```python
from build123d import *

# Parameters (mm, degrees)
F1_DEPTH = 40.2336
F2_DEPTH = 15.7734
F3_R     = 3.302


# Not quite as in the source:
# - a feature names something its author has since deleted; it is built from what else it names


with BuildPart() as f1:
    # F0 (on Top) → F1 (new body)
    with BuildSketch(Plane.XY):
        with BuildLine():
            ThreePointArc((5.2118165727, -28.0956863773), (21.9710978739, -18.2702348977), (28.575, 0))
            ThreePointArc((28.575, 0), (21.9710978739, 18.2702348977), (5.2118165727, 28.0956863773))
            ThreePointArc((5.2118165727, 28.0956863773), (-28.575, 0), (5.2118165727, -28.0956863773))
        make_face()
        with BuildLine():
            ThreePointArc((13.4477648793, -4.826), (-14.2875, 0), (13.4477648793, 4.826))
            Line((13.4477648793, 4.826), (19.7977648793, 4.826))
            Line((19.7977648793, 4.826), (19.7977648793, 0))
            Line((19.7977648793, 0), (19.7977648793, -4.826))
            Line((19.7977648793, -4.826), (13.4477648793, -4.826))
        make_face(mode=Mode.SUBTRACT)
    extrude(amount=F1_DEPTH)

    # F0 (on Top) → F2 (join)
    with BuildSketch(Plane.XY):
        with BuildLine():
            ThreePointArc((5.2118165727, 28.0956863773), (21.9710978739, 18.2702348977), (28.575, 0))
            Line((28.575, 0), (34.925, 0))
            ThreePointArc((34.925, 0), (40.5046158184, 13.4703841816), (53.975, 19.05))
            Line((53.975, 19.05), (5.2118165727, 28.0956863773))
        make_face()
        with BuildLine():
            Line((34.925, 0), (28.575, 0))
            ThreePointArc((28.575, 0), (21.9710978739, -18.2702348977), (5.2118165727, -28.0956863773))
            Line((5.2118165727, -28.0956863773), (53.975, -19.05))
            ThreePointArc((53.975, -19.05), (40.5046158184, -13.4703841816), (34.925, 0))
        make_face()
        with BuildLine():
            ThreePointArc((53.975, 19.05), (40.5046158184, 13.4703841816), (34.925, 0))
            ThreePointArc((34.925, 0), (40.5046158184, -13.4703841816), (53.975, -19.05))
            ThreePointArc((53.975, -19.05), (67.4453841816, -13.4703841816), (73.025, 0))
            ThreePointArc((73.025, 0), (67.4453841816, 13.4703841816), (53.975, 19.05))
        make_face()
        with BuildLine():
            ThreePointArc((64.135, 0), (53.975, -10.16), (43.815, 0))
            ThreePointArc((43.815, 0), (53.975, 10.16), (64.135, 0))
        make_face(mode=Mode.SUBTRACT)
    extrude(amount=F2_DEPTH)

    # F3
    f3_edges = [f1.edges().sort_by_distance(p)[0] for p in [
        (-5.211817, 28.095686, 40.2336),
    ]]
    fillet(f3_edges, radius=F3_R)


solid = f1.part
```
Read the model definition and answer for the solid it produces. Units are mm, in the model's axes. A direction names the side the tool comes from. Coordinates: 2 decimals unless noted, no trailing zeros. Write each loop counter-clockwise with the first axis right and the second up, starting at its lowest first coordinate (ties: lowest second). Pieces come first, ordered by that corner, then holes. Notation, with made-up numbers: (80.25, 77) - (89.25, 77) arc R30 cw to (89.25, 108) - close; hole circle Ø10 at (67.5, -15). An arc over 180 degrees is marked (long way). Answer as a JSON object with one key per item and string values. Group by question number.
1. Which of the six approach directions +Z, -Z, +X, -X, +Y, -Y give full straight-line access (tool end or side, diameter ignored) to faces 4 (the flat face through (22, 0, 0)), 5 (the flat face through (19.798, 0, 20))?
2. Consider L1, parallel to Y at x = 0, z = 22 (1 decimal); L2, parallel to X at y = 0, z = 18 (1 decimal); L3, parallel to X at y = 3, z = 15.5. Determine where each line is inside the solid, lowest interval first. Write a range as [from, to].
3. Each of these flat-tipped pins is pushed along its axis until it touches: P1, Ø5, axis at x = 16, z = 24, coming from the +Y side; P2, Ø10, axis at x = 55.5, y = 8, coming from the +Z side; P3, Ø1.5, axis at y = 19, z = 7, coming from the -X side; P4, Ø12, axis at x = 51, y = 19.5, coming from the -Z side. Where does it stop, or does it pass through?
4. A cutting plane is placed at C-C (x = 66.5). Determine the outline of the cut face in (y, z), plus the area to 3 significant figures.
5. The mould has two halves that part along X. Classify faces 1 (the flat face through (39, 0, 15.773)), 2 (the cylindrical face through (44.3, 3.1, 7.8)), 3 (the flat face through (29.93, 23.51, 7.78)): +X half, -X half, draft (parallel to the pull), parting line (faces both ways), or undercut.
6. A cutting plane is placed at B-B (z = 11). Give the number of separate pieces and of enclosed holes in the cut face, plus the area to 3 significant figures.
Worked out:
{
 "1": {"face 4": "-Z, +X, -X, +Y, -Y", "face 5": "+Z, -Z"},
 "2": {"L1": "y = [-28.6, -14.3], [14.3, 28.6]", "L2": "x = [-28.6, -14.3], [19.8, 28.6]", "L3": "x = [-28.42, -13.97], [19.8, 44.27], [63.68, 72.79]"},
 "3": {"P1": "stops at y = 25.18", "P2": "stops at z = 15.77", "P3": "stops at x = -21.99", "P4": "stops at z = 0"},
 "4": {"outline": "(-14.35, 0) - (14.35, 0) - (14.35, 15.77) - (-14.35, 15.77) - close", "area": "453 mm²"},
 "5": {"face 1": "draft", "face 2": "undercut", "face 3": "+X half"},
 "6": {"separate pieces": "1", "enclosed holes": "2", "area": "3,430 mm²"}
}
